Here's how the part is built. I have some questions about the finished solid (model axes, mm). Coordinates: 2 decimals unless noted, no trailing zeros. Order: outer loops, then holes, each group sorted by start corner. A loop starts at its lowest first (then second) coordinate and runs counter-clockwise, first axis right, second up. Notation, with made-up numbers: (54, 1) - (97, 1) arc R17 cw to (97, 19) - close; hole circle Ø7 at (8, 73.5). An arc over 180 degrees is marked (long way). Answer as CSV lines item,"result". Start each with the question number.
Q1. Suppose I cut it at B-B (z = 2.45). Please give me the cut outline in (x, y).
Q2. Suppose I cut it at A-A (y = 0). Please give me the cut outline in (x, z), then the cut area to 3 significant figures.
Q3. I need wall thicknesses on line 1 (X direction, y = -0.25, z = 2.6); line 2 (X direction, y = 1.75, z = 2.6); line 3 (Y direction, x = -35, z = 2.3). Which ranges of each line are inside material? Lowest first, please.
from build123d import *

# Parameters (mm, degrees)
SKETCH_1_W          = 95
SKETCH_1_H          = 13
EXTRUDE_1_DEPTH     = 3
SKETCH_2_R          = 4
CUT_EXTRUDE_1_DEPTH = 3
FILLET_1_R          = 3
SKETCH_3_R          = 4
CUT_EXTRUDE_2_DEPTH = 3
SKETCH_4_W          = 4.5
SKETCH_4_H          = 8
CUT_EXTRUDE_3_DEPTH = 3


with BuildPart() as part:
    # ｽｹｯﾁ1 → ﾎﾞｽ - 押し出し1 (new body)
    with BuildSketch(Plane.XY):
        Rectangle(SKETCH_1_W, SKETCH_1_H)
    extrude(amount=EXTRUDE_1_DEPTH)

    # ｽｹｯﾁ2 → ｶｯﾄ - 押し出し1 (cut)
    with BuildSketch(Plane.XY.offset(3)):
        with Locations((41, 0)):
            Circle(SKETCH_2_R)
        with Locations((-41, 0)):
            Circle(SKETCH_2_R)
    extrude(amount=-CUT_EXTRUDE_1_DEPTH, mode=Mode.SUBTRACT)

    # ﾌｨﾚｯﾄ1
    fillet_1_edges = [part.edges().sort_by_distance(p)[0] for p in [
        (47.5, -6.5, 1.5),
        (-47.5, -6.5, 1.5),
        (-47.5, 6.5, 1.5),
        (47.5, 6.5, 1.5),
    ]]
    fillet(fillet_1_edges, radius=FILLET_1_R)

    # ｽｹｯﾁ3 → ｶｯﾄ - 押し出し2 (cut)
    with BuildSketch(Plane.XY.offset(3)):
        with Locations((36.5, 0)):
            Circle(SKETCH_3_R)
        with Locations((-36.5, 0)):
            Circle(SKETCH_3_R)
    extrude(amount=-CUT_EXTRUDE_2_DEPTH, mode=Mode.SUBTRACT)

    # ｽｹｯﾁ4 → ｶｯﾄ - 押し出し3 (cut)
    with BuildSketch(Plane.XY.offset(3)):
        with Locations((-38.75, 0)):
            Rectangle(SKETCH_4_W, SKETCH_4_H)
        with Locations((38.75, 0)):
            Rectangle(SKETCH_4_W, SKETCH_4_H)
    extrude(amount=-CUT_EXTRUDE_3_DEPTH, mode=Mode.SUBTRACT)


solid = part.part
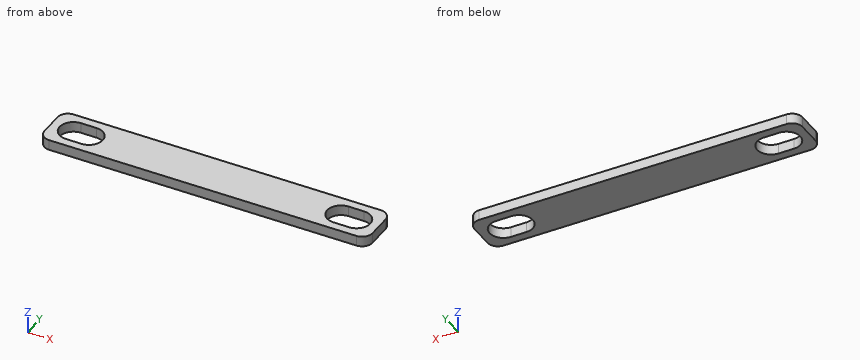
Here are the results:
1,outline,"(-47.5, -3.5) arc R3 ccw to (-44.5, -6.5) - (44.5, -6.5) arc R3 ccw to (47.5, -3.5) - (47.5, 3.5) arc R3 ccw to (44.5, 6.5) - (-44.5, 6.5) arc R3 ccw to (-47.5, 3.5) - close; hole (-41, -4) - (-36.5, -4) arc R4 ccw to (-36.5, 4) - (-41, 4) arc R4 ccw to start; hole (36.5, -4) - (41, -4) arc R4 ccw to (41, 4) - (36.5, 4) arc R4 ccw to start"
2,outline,"(-47.5, 0) - (-45, 0) - (-45, 3) - (-47.5, 3) - close; (-32.5, 0) - (32.5, 0) - (32.5, 3) - (-32.5, 3) - close; (45, 0) - (47.5, 0) - (47.5, 3) - (45, 3) - close"
2,area,"210 mm²"
3,line 1,"x = -47.5 to -44.99, -32.51 to 32.51, 44.99 to 47.5"
3,line 2,"x = -47.5 to -44.6, -32.9 to 32.9, 44.6 to 47.5"
3,line 3,"y = -6.5 to -3.71, 3.71 to 6.5"
